Part print with two shaded views. Sizes in mm from the minimum x, y, z corner. Round coordinates to 2 decimals unless told otherwise and drop trailing zeros. Write each loop counter-clockwise with the first axis right and the second up, starting at its lowest first coordinate (ties: lowest second). Pieces come first, ordered by that corner, then holes. Notation, with made-up numbers: (52.25, 23) -> (77.25, 23) arc R12 cw to (77.25, 44) -> close; hole circle Ø7 at (54.5, -7.75). An arc over 180 degrees is marked (long way). Return JSON: item names as keys, results as strings.
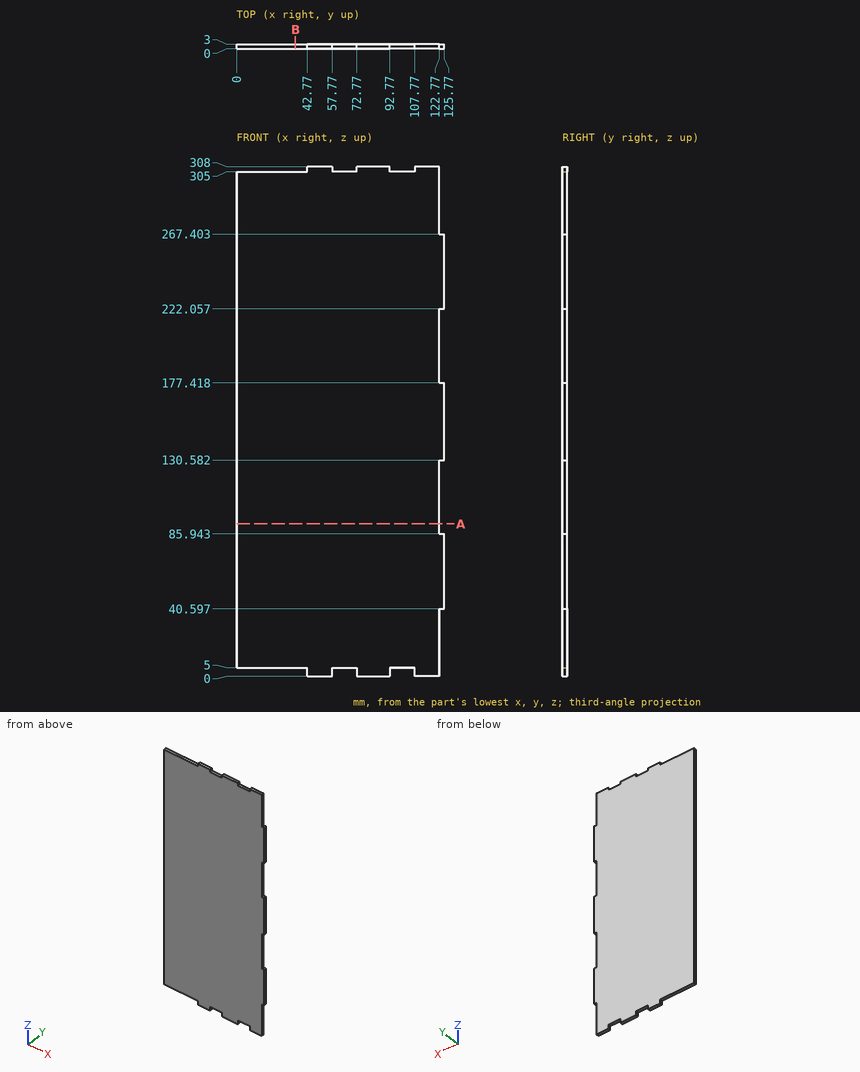
Q1. Saw through at A-A on z = 92. List the corners of the cut face in (x, y), then the cut area to 3 significant figures.
Verdict:
{"outline": "(0, 0) -> (122.77, 0) -> (122.77, 3) -> (0, 3) -> close", "area": "368 mm²"}
Q2. Wall check: L1, parallel to X at y = 1.1, z = 12; L2, parallel to Z at x = 10, y = 0.45. Give the ranges that are in metal, low to high.
Verdict:
{"L1": "x = 0 to 122.77", "L2": "z = 5 to 305"}
Q3. Saw through at B-B on x = 35.5. List the corners of the cut face in (y, z), then the cut area to 3 significant figures.
Verdict:
{"outline": "(0, 5) -> (3, 5) -> (3, 305) -> (0, 305) -> close", "area": "900 mm²"}
Q4. Pin check, flat tips, straight feed: pin 1 Ø0.9 at (x, y) = (97, 1.5) entering from -Z; pin 2 Ø0.9 at (y, z) = (1.5, 2) entering from -X; pin 3 Ø0.9 at (x, y) = (124, 2) entering from +Z. Stop position of each tip, or through.
Verdict:
{"pin 1": "stops at z = 5", "pin 2": "stops at x = 42.77", "pin 3": "stops at z = 267.4"}
